```python
from build123d import *

# Parameters (mm, degrees)
ESBO_O1_W                = 13.1
ESBO_O1_H                = 21
RESSALTO_EXTRUS_O1_DEPTH = 15
ESBO_O2_W                = 15
ESBO_O2_H                = 3
RESSALTO_EXTRUS_O2_DEPTH = 10
ESBO_O3_W                = 3
ESBO_O3_H                = 8
RESSALTO_EXTRUS_O3_DEPTH = 10
CORTE_EXTRUS_O1_DEPTH    = 19
ESBO_O5_R                = 1.5
CORTE_EXTRUS_O2_DEPTH    = 19
RESSALTO_EXTRUS_O4_DEPTH = 10
CORTE_EXTRUS_O3_DEPTH    = 23
ESBO_O8_R                = 1.5
CORTE_EXTRUS_O4_DEPTH    = 23


with BuildPart() as part:
    # Esboço1 → Ressalto-extrusão1 (new body)
    with BuildSketch(Plane.XY):
        Polygon((0, 26), (5, 26), (5, -5), (-18.1, -5), (-18.1, 0), (-18.1, 26), align=None)
        with Locations((-6.55, 10.5)):
            Rectangle(ESBO_O1_W, ESBO_O1_H, mode=Mode.SUBTRACT)
    extrude(amount=RESSALTO_EXTRUS_O1_DEPTH)

    # Esboço2 → Ressalto-extrusão2 (add)
    with BuildSketch(Plane.ZY.offset(18.1)):
        with Locations((7.5, -3.5)):
            Rectangle(ESBO_O2_W, ESBO_O2_H)
    extrude(amount=RESSALTO_EXTRUS_O2_DEPTH)

    # Esboço3 → Ressalto-extrusão3 (add)
    with BuildSketch(Plane.ZY.offset(18.1)):
        with Locations((1.5, 2)):
            Rectangle(ESBO_O3_W, ESBO_O3_H)
        with Locations((13.5, 2)):
            Rectangle(ESBO_O3_W, ESBO_O3_H)
    extrude(amount=RESSALTO_EXTRUS_O3_DEPTH)

    # Esboço4 → Corte-extrusão1 (cut)
    with BuildSketch(Plane(origin=(0, 0, 0), x_dir=(-1, 0, 0), z_dir=(0, 0, -1))):
        Polygon((18.1, 6), (28.1, -2), (28.1, 6), align=None)
    extrude(amount=-CORTE_EXTRUS_O1_DEPTH, mode=Mode.SUBTRACT)

    # Esboço5 → Corte-extrusão2 (cut)
    with BuildSketch(Plane(origin=(0, -2, 0), x_dir=(1, 0, 0), z_dir=(0, 1, 0))):
        with Locations(Location((-23.1, -7.5, 0), (0, 0, 270))):
            Circle(ESBO_O5_R)
    extrude(amount=-CORTE_EXTRUS_O2_DEPTH, mode=Mode.SUBTRACT)

    # Esboço6 → Ressalto-extrusão4 (add)
    with BuildSketch(Plane(origin=(5, 0, 0), x_dir=(0, 0, -1), z_dir=(1, 0, 0))):
        Polygon((-15, -5), (-15, 8.409277905), (-12, 8.409277905), (-12, -2), (-3, -2), (-3, 8.409277905), (0, 8.409277905), (0, -5), align=None)
    extrude(amount=RESSALTO_EXTRUS_O4_DEPTH)

    # Esboço7 → Corte-extrusão3 (cut)
    with BuildSketch(Plane(origin=(0, 0, 0), x_dir=(-1, 0, 0), z_dir=(0, 0, -1))):
        Polygon((-5, 8.409277905), (-15, -2), (-15, 8.409277905), align=None)
    extrude(amount=-CORTE_EXTRUS_O3_DEPTH, mode=Mode.SUBTRACT)

    # Esboço8 → Corte-extrusão4 (cut)
    with BuildSketch(Plane(origin=(0, -2, 0), x_dir=(1, 0, 0), z_dir=(0, 1, 0))):
        with Locations(Location((10, -7.5, 0), (0, 0, 270))):
            Circle(ESBO_O8_R)
    extrude(amount=-CORTE_EXTRUS_O4_DEPTH, mode=Mode.SUBTRACT)


solid = part.part
```
Check sheet for the modelled part. Datum: model origin and axes. Units: mm. A direction names the side the tool comes from. Round coordinates to 2 decimals unless told otherwise and drop trailing zeros. Order: outer loops, then holes, each group sorted by start corner. A loop starts at its lowest first (then second) coordinate and runs counter-clockwise, first axis right, second up.
1) Section check D-D (z = 2). Record the boundary of the cut face in (x, y).
2) Section check B-B (x = -23.1). Record the boundary of the cut face in (y, z), and give its area (3 significant figures).
3) Mould release check, pull along Z, two halves, no side actions. Record for faces 1 (the flat face through (9, 2, 3)), 2 (the flat face through (0, 10, 7)), 3 (the flat face through (3, 7, 15)), 4 (the flat face through (3, 7, 0)): +Z half, -Z half, draft (parallel to the pull), parting line (faces both ways), or undercut.
4) Section check A-A (z = 7.5). Record the boundary of the cut face in (x, y).
5) Tool access check on faces 5 (the flat face through (-22, -2, 6)), 6 (the flat face through (9.93, 3.28, 13.48)), 7 (the flat face through (5, 15, 7)), 8 (the cylindrical face through (9.1, -3.5, 6.3)), 9 (the flat face through (-13.1, 10, 7)). Record the directions out of +Z, -Z, +X, -X, +Y, -Y that give a thin tool (end or side, any length) a straight path to the whole face; none if there is none.
6) Section check C-C (y = 20). Record the boundary of the cut face in (x, z).
7) Go/stop test with flat-tipped pins: pin 1 Ø4 at (y, z) = (12.5, 5.5) entering from +X; pin 2 Ø3 at (y, z) = (1.5, 12) entering from -X; pin 3 Ø4.5 at (y, z) = (7, 4.5) entering from +X (3 decimals); pin 4 Ø1 at (x, y) = (-19, 19.5) entering from +Z. Record where each tip stops, or that it passes through.
8) Scan lines: line 1 (X direction, y = -4.05, z = 7.5); line 2 (Y direction, x = -6.5, z = 4.5); line 3 (Z direction, x = -23, y = -3). Record each from-to range of solid material in increasing order.
Result:
1. outline: (-28.1, -5) - (15, -5) - (15, -2) - (5, 8.41) - (5, 26) - (-18.1, 26) - (-18.1, 6) - (-28.1, -2) - close; hole (-13.1, 0) - (0, 0) - (0, 21) - (-13.1, 21) - close
2. outline: (-5, 0) - (2, 0) - (2, 3) - (-2, 3) - (-2, 6) - (-5, 6) - close; (-5, 9) - (-2, 9) - (-2, 12) - (2, 12) - (2, 15) - (-5, 15) - close
2. area: 60.0 mm2
3. face 1: undercut
3. face 2: draft
3. face 3: +Z half
3. face 4: -Z half
4. outline: (-28.1, -5) - (-24.6, -5) - (-24.6, -2) - (-28.1, -2) - close; (-21.6, -5) - (8.5, -5) - (8.5, -2) - (5, -2) - (5, 26) - (-18.1, 26) - (-18.1, -2) - (-21.6, -2) - close; (11.5, -5) - (15, -5) - (15, -2) - (11.5, -2) - close; hole (-13.1, 0) - (0, 0) - (0, 21) - (-13.1, 21) - close
5. face 5: -X, +Y
5. face 6: +Z, -Z, +X, +Y
5. face 7: +X, +Y
5. face 8: +Y, -Y
5. face 9: +Z, -Z
6. outline: (-18.1, 0) - (-13.1, 0) - (-13.1, 15) - (-18.1, 15) - close; (0, 0) - (5, 0) - (5, 15) - (0, 15) - close
7. pin 1: stops at x = 5
7. pin 2: stops at x = -25.6
7. pin 3: stops at x = 7.965
7. pin 4: passes through
8. line 1: x = -28.1 to -24.6, -21.6 to 8.5, 11.5 to 15
8. line 2: y = -5 to 0, 21 to 26
8. line 3: z = 0 to 6, 9 to 15
